Could you check a few things on this model? Use its own coordinates, in mm. A direction names the side the tool comes from. Give positions to 0.01 mm unless a question says otherwise; leave off trailing zeros. Order: outer loops, then holes, each group sorted by start corner. A loop starts at its lowest first (then second) coordinate and runs counter-clockwise, first axis right, second up.
(1) Will these pins go through, and if not, where does the flat tip stop? pin 1 (2 mm diameter, centred on y = 3.5, z = 20.5, fed in from +X); pin 2 (1.6 mm diameter, centred on y = -2, z = 0.5, fed in from +X); pin 3 (12 mm diameter, centred on x = -17.5, z = -32.5, fed in from -Y); pin 4 (6.5 mm diameter, centred on x = 40, y = -3, fed in from -Z) (3 decimals).
(2) Imagine slicing it at D-D, the plane x = 0. Write out the boundary of the cut face in (y, z).
(3) If I drill on probe 1 along Z at (x, y) = (-0.5, -2.25); probe 2 along X at (y, z) = (-2.5, -5); probe 3 along Z at (x, y) = (40, -3.5) (1 decimal), over which ranges is the centre line in solid material (lowest first)?
(4) If we mould it in two halves opening along Z, with no side actions, what happens to faces 5 (the cylindrical face through (-25.4, 0.1, 0.2)), 6 (the cylindrical face through (-2.897, 0.089, -25.783)), 7 (the flat face through (-13, -6.35, 3))? For each: released by +Z, released by -Z, zero draft, split by the parting line, or undercut.
(5) Imagine slicing it at C-C, the plane y = 0. State how many separate pieces and enclosed holes the cut face has, then the cut area to 3 significant figures.
(6) Imagine slicing it at B-B, the plane z = -7. Write out the boundary of the cut face in (x, y) (3 decimals), then the cut area to 3 significant figures.
(7) On a 3-axis mill with a long thin cutter (end or side, diameter ignored), from which of +Z, -Z, +X, -X, +Y, -Y can I reach the whole of each face in a straight line? I mean faces 1 (the flat face through (42, 0, -4.762)), 2 (the flat face through (-25.43, 2.91, -26.16)), 3 (the flat face through (-16.234, 0.089, -39.029)), 4 (the flat face through (-11.67, -1.32, -40.62)). Say none if no direction works.
from build123d import *

# Parameters (mm, degrees)
SKETCH1_R                             = 12.7
SKETCH1_R_2                           = 1.8288
BOSS_EXTRUDE1_DEPTH                   = 6.35
F_1_4_0_25_DIAMETER_HOLE1_D           = 6.35
F_1_4_0_25_DIAMETER_HOLE1_ON_FACE_2_D = 6.35
F_1_4_0_25_DIAMETER_HOLE1_ON_FACE_3_D = 6.35
F_1_4_0_25_DIAMETER_HOLE1_ON_FACE_4_D = 6.35
F_1_4_0_25_DIAMETER_HOLE1_ON_FACE_5_D = 6.35
F_1_4_0_25_DIAMETER_HOLE1_ON_FACE_6_D = 6.35
FILLET1_R                             = 3.175


with BuildPart() as part:
    # Sketch1 → Boss-Extrude1 (new, symmetric)
    with BuildSketch(Plane(origin=(0, 0, 0), x_dir=(1, 0, 0), z_dir=(0, 1, 0))):
        with BuildLine():
            Line((25.4, 4.7625), (25.4, -4.7625))
            Line((25.4, -4.7625), (50.8, -4.7625))
            Line((50.8, -4.7625), (50.8, -9.525))
            Line((50.8, -9.525), (23.546430197, -9.525))
            ThreePointArc((23.546430197, -9.525), (12.881044339, -21.891521115), (-3.108809324, -25.209032202))
            Line((-3.108809324, -25.209032202), (-16.344312849, -49.032938546))
            Line((-16.344312849, -49.032938546), (-20.507486876, -46.720064087))
            Line((-20.507486876, -46.720064087), (-8.172156424, -24.516469273))
            Line((-8.172156424, -24.516469273), (-16.498504479, -19.890720354))
            Line((-16.498504479, -19.890720354), (-28.833834931, -42.094315167))
            Line((-28.833834931, -42.094315167), (-32.997008959, -39.781440707))
            Line((-32.997008959, -39.781440707), (-19.761505434, -15.957534364))
            ThreePointArc((-19.761505434, -15.957534364), (-25.4, 0), (-19.761505434, 15.957534364))
            Line((-19.761505434, 15.957534364), (-32.997008959, 39.781440707))
            Line((-32.997008959, 39.781440707), (-28.833834931, 42.094315167))
            Line((-28.833834931, 42.094315167), (-16.498504479, 19.890720354))
            Line((-16.498504479, 19.890720354), (-8.172156424, 24.516469273))
            Line((-8.172156424, 24.516469273), (-20.507486876, 46.720064087))
            Line((-20.507486876, 46.720064087), (-16.344312849, 49.032938546))
            Line((-16.344312849, 49.032938546), (-3.108809324, 25.209032202))
            ThreePointArc((-3.108809324, 25.209032202), (12.881044339, 21.891521115), (23.546430197, 9.525))
            Line((23.546430197, 9.525), (50.8, 9.525))
            Line((50.8, 9.525), (50.8, 4.7625))
            Line((50.8, 4.7625), (25.4, 4.7625))
        make_face()
        with Locations(Location((0, 0, 0), (0, 0, 270))):
            Circle(SKETCH1_R, mode=Mode.SUBTRACT)
        with Locations(Location((-13.470384182, 13.470384182, 0), (0, 0, 270))):
            Circle(SKETCH1_R_2, mode=Mode.SUBTRACT)
        with Locations(Location((13.470384182, 13.470384182, 0), (0, 0, 270))):
            Circle(SKETCH1_R_2, mode=Mode.SUBTRACT)
        with Locations(Location((13.470384182, -13.470384182, 0), (0, 0, 270))):
            Circle(SKETCH1_R_2, mode=Mode.SUBTRACT)
        with Locations(Location((-13.470384182, -13.470384182, 0), (0, 0, 270))):
            Circle(SKETCH1_R_2, mode=Mode.SUBTRACT)
    extrude(amount=BOSS_EXTRUDE1_DEPTH, both=True)

    # 1/4 (0.25) Diameter Hole1 (through all)
    with Locations(Plane(origin=(38.1, 0, -4.7625), x_dir=(0, 1, 0), z_dir=(0, 0, 1))):
        with Locations((0, 0)):
            Hole(F_1_4_0_25_DIAMETER_HOLE1_D / 2)

    # 1/4 (0.25) Diameter Hole1 on face 2 (through all)
    with Locations(Plane(origin=(-14.33982165, 0, -35.61826668), x_dir=(-0.48564310099, 0, -0.874157181782), z_dir=(-0.874157181782, 0, 0.48564310099))):
        with Locations((0, 0)):
            Hole(F_1_4_0_25_DIAMETER_HOLE1_ON_FACE_2_D / 2)

    # 1/4 (0.25) Diameter Hole1 on face 3 (through all)
    with Locations(Plane(origin=(-22.666169705, 0, 30.99251776), x_dir=(-0.48564310099, 0, 0.874157181782), z_dir=(0.874157181782, 0, 0.48564310099))):
        with Locations((1e-09, 0)):
            Hole(F_1_4_0_25_DIAMETER_HOLE1_ON_FACE_3_D / 2)

    # 1/4 (0.25) Diameter Hole1 on face 4 (through all)
    with Locations(Plane(origin=(-14.33982165, 0, 35.61826668), x_dir=(0.48564310099, 0, -0.874157181782), z_dir=(-0.874157181782, 0, -0.48564310099))):
        with Locations((0, 0)):
            Hole(F_1_4_0_25_DIAMETER_HOLE1_ON_FACE_4_D / 2)

    # 1/4 (0.25) Diameter Hole1 on face 5 (through all)
    with Locations(Plane(origin=(-22.666169705, 0, -30.99251776), x_dir=(0.48564310099, 0, 0.874157181782), z_dir=(0.874157181782, 0, -0.48564310099))):
        with Locations((-1e-09, 0)):
            Hole(F_1_4_0_25_DIAMETER_HOLE1_ON_FACE_5_D / 2)

    # 1/4 (0.25) Diameter Hole1 on face 6 (through all)
    with Locations(Plane(origin=(38.1, 0, 4.7625), x_dir=(-1, 0, 0), z_dir=(0, 0, -1))):
        with Locations((0, 0)):
            Hole(F_1_4_0_25_DIAMETER_HOLE1_ON_FACE_6_D / 2)

    # Fillet1
    fillet1_edges = [part.edges().sort_by_distance(p)[0] for p in [
        (25.4, 0, -4.7625),
        (25.4, 0, 4.7625),
        (23.546430197, 0, 9.525),
        (-3.108809324, 0, 25.209032202),
        (-8.172156424, 0, 24.516469273),
        (-16.498504479, 0, 19.890720354),
        (-19.761505434, 0, 15.957534364),
        (-19.761505434, 0, -15.957534364),
        (-16.498504479, 0, -19.890720354),
        (-8.172156424, 0, -24.516469273),
        (-3.108809324, 0, -25.209032202),
        (23.546430197, 0, -9.525),
    ]]
    fillet(fillet1_edges, radius=FILLET1_R)


solid = part.part
Answer block:
1. pin 1: stops at x = 16.28
1. pin 2: stops at x = 25.4
1. pin 3: stops at y = -6.35
1. pin 4: stops at z = -9.525
2. outline: (-6.35, -25.4) - (6.35, -25.4) - (6.35, -12.7) - (-6.35, -12.7) - close; (-6.35, 12.7) - (6.35, 12.7) - (6.35, 25.4) - (-6.35, 25.4) - close
3. probe 1: z = -25.4 to -12.69, 12.69 to 25.4
3. probe 2: x = -24.9 to -11.67, 11.67 to 36.14, 40.06 to 50.8
3. probe 3: z = -9.5 to -4.8, 4.8 to 9.5
4. face 5: undercut
4. face 6: released by -Z
4. face 7: zero draft
5. separate pieces: 7
5. enclosed holes: 5
5. area: 2,070 mm2
6. outline: (-24.416, -6.35) - (-10.597, -6.35) - (-10.597, 6.35) - (-24.416, 6.35) - close; (10.597, -6.35) - (50.8, -6.35) - (50.8, 6.35) - (10.597, 6.35) - close; hole circle Ø6.35 at (38.1, 0)
6. area: 654 mm2
7. face 1: +X, +Y, -Y
7. face 2: -X, +Y, -Y
7. face 3: +Y, -Y
7. face 4: -Z, +X, +Y, -Y
